Here's the drawing with two shaded views (mm, measured from the low corner). I have some questions. Coordinates: 2 decimals unless noted, no trailing zeros. Write each loop counter-clockwise with the first axis right and the second up, starting at its lowest first coordinate (ties: lowest second). Pieces come first, ordered by that corner, then holes. Notation, with made-up numbers: (75, 7.25) -> (100, 7.25) arc R31 ccw to (100, 35.25) -> close; hole circle Ø6 at (54.25, -21). An arc over 180 degrees is marked (long way). Put each result on its own line as item: value.
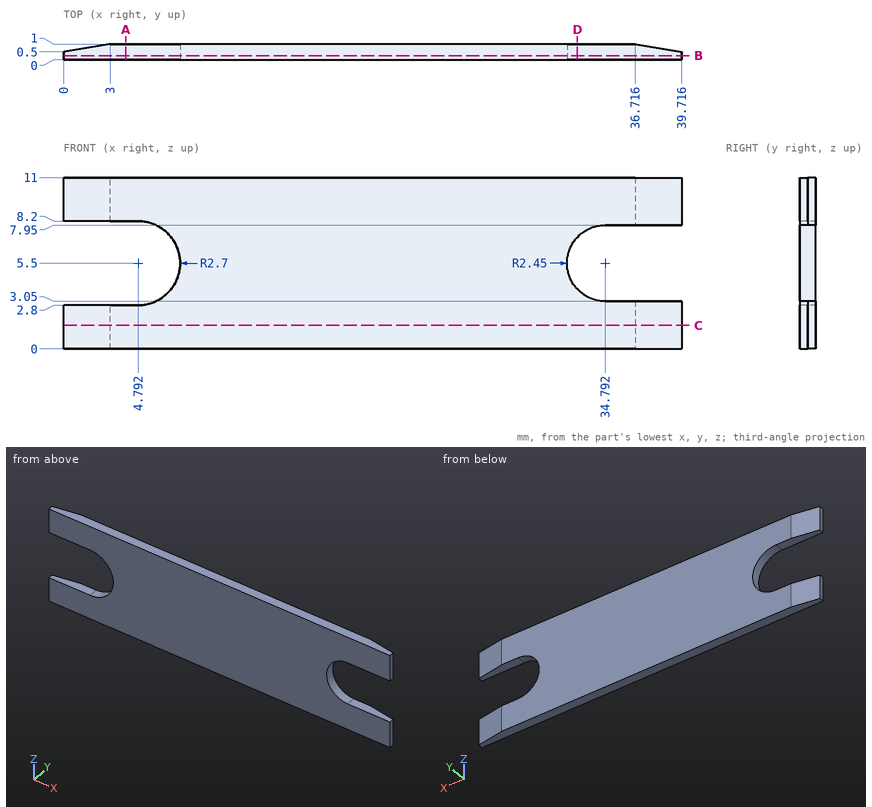
Item 1: Imagine slicing it at D-D on x = 33. Write out the boundary of the cut face in (y, z).
Output:
outline: (0, 0) -> (1, 0) -> (1, 3.83) -> (0, 3.83) -> close; (0, 7.17) -> (1, 7.17) -> (1, 11) -> (0, 11) -> close
Item 2: Imagine slicing it at B-B on y = 0.25. Write out the boundary of the cut face in (x, z), then the cut area to 3 significant figures.
Output:
outline: (0, 0) -> (39.72, 0) -> (39.72, 3.05) -> (34.79, 3.05) arc R2.45 cw to (34.79, 7.95) -> (39.72, 7.95) -> (39.72, 11) -> (0, 11) -> (0, 8.2) -> (4.79, 8.2) arc R2.7 cw to (4.79, 2.8) -> (0, 2.8) -> close
area: 366 mm²
Item 3: Imagine slicing it at C-C on z = 1.5. Write out the boundary of the cut face in (x, y).
Output:
outline: (0, 0) -> (39.72, 0) -> (39.72, 0.5) -> (36.72, 1) -> (3, 1) -> (0, 0.5) -> close
Item 4: Imagine slicing it at A-A on x = 4. Write out the boundary of the cut face in (y, z).
Output:
outline: (0, 0) -> (1, 0) -> (1, 2.8) -> (0, 2.8) -> close; (0, 8.2) -> (1, 8.2) -> (1, 11) -> (0, 11) -> close
Item 5: Please list where these lines run through material, in increasing order: line 1 along Z through (x, y) = (2, 0.1); line 2 along Z through (x, y) = (33, 0.85); line 3 along X through (y, z) = (0.3, 7) (1 decimal). Write a range as from..to.
Output:
line 1: z = 0..2.8, 8.2..11
line 2: z = 0..3.83, 7.17..11
line 3: x = 7..32.9
